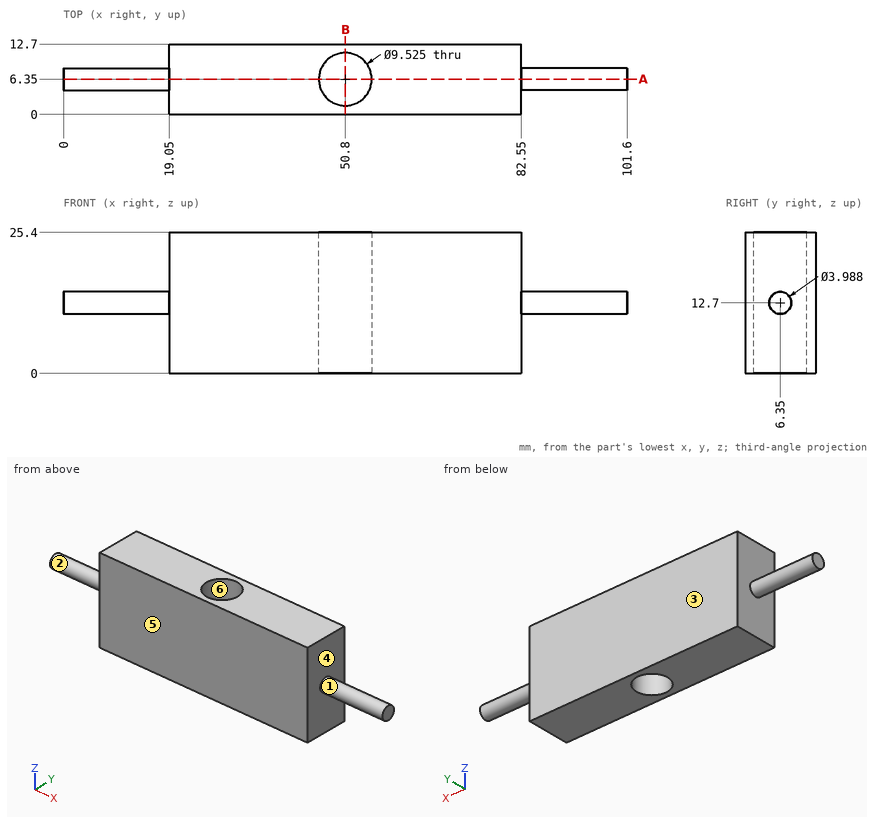
Source: three-view drawing plus pictorial views. Frame: mm from the lowest corner of the part. A direction names the side the tool comes from. Give positions to 0.01 mm unless a question says otherwise; leave off trailing zeros. Order: outer loops, then holes, each group sorted by start corner. A loop starts at its lowest first (then second) coordinate and runs counter-clockwise, first axis right, second up. Notation, with made-up numbers: (22.25, 43.25) -> (50.25, 43.25) arc R21 cw to (50.25, 59.25) -> close; hole circle Ø9 at (-24, -39.75). An arc over 180 degrees is marked (long way). Use a Markdown table: item, result.
Q1. Section B-B (x = 50.8). Return the cut outline in (y, z).
A:
| item | result |
|---|---|
| outline | (0, 0) -> (1.59, 0) -> (1.59, 25.4) -> (0, 25.4) -> close; (11.11, 0) -> (12.7, 0) -> (12.7, 25.4) -> (11.11, 25.4) -> close |
Q2. First-contact query: P1, Ø1, axis at x = 10.5, y = 6.5, coming from the -Z side; P2, Ø2, axis at x = 10.5, y = 9, coming from the +Z side; P3, Ø1, axis at y = 7.5, z = 8, coming from the +X side. Flat tips, straight axial feed; report the tip coordinate or a pass-through.
A:
| item | result |
|---|---|
| P1 | z = 10.71 |
| P2 | z = 13.82 |
| P3 | x = 82.55 |
Q3. Pull-direction query (X, two-part tool) for the marked faces 4, 5 and 6; classes: +X half, -X half, draft (parallel to the pull), parting line (faces both ways), or undercut.
A:
| item | result |
|---|---|
| face 4 | +X half |
| face 5 | draft |
| face 6 | undercut |
Q4. Material intervals for line 1 (Y direction, x = 50.8, z = 14.25); line 2 (X direction, y = 7, z = 23); line 3 (X direction, y = 8.25, z = 5.75), sorted ascending. Write a range as [from, to].
A:
| item | result |
|---|---|
| line 1 | [0, 1.59], [11.11, 12.7] |
| line 2 | [19.05, 46.08], [55.52, 82.55] |
| line 3 | [19.05, 46.43], [55.17, 82.55] |
Q5. Section A-A (y = 6.35). Return the cut outline in (x, z).
A:
| item | result |
|---|---|
| outline | (0, 10.71) -> (19.05, 10.71) -> (19.05, 0) -> (46.04, 0) -> (46.04, 25.4) -> (19.05, 25.4) -> (19.05, 14.69) -> (0, 14.69) -> close; (55.56, 0) -> (82.55, 0) -> (82.55, 10.71) -> (101.6, 10.71) -> (101.6, 14.69) -> (82.55, 14.69) -> (82.55, 25.4) -> (55.56, 25.4) -> close |
Q6. Access query for the marked faces 1, 2 and 3. Directions: +Z, -Z, +X, -X, +Y, -Y. A direction counts if a zero-diameter tool reaches every point of the face in a straight line with its end or side. Return the directions, or none.
A:
| item | result |
|---|---|
| face 1 | +X |
| face 2 | -X |
| face 3 | +Z, -Z, +X, -X, +Y |
